Geometry check sheet. Reference: the model listing, model coordinates, mm. A direction names the side the tool comes from. Give positions to 0.01 mm unless a question says otherwise; leave off trailing zeros. Write item = value, one per line. Start each with the question number.
1. Depth check by flat-ended pin: P1, Ø4, axis at x = -1.5, z = -34, coming from the -Y side; P2, Ø1.3, axis at y = -2, z = -67, coming from the +X side; P3, Ø1.3, axis at x = -1.5, z = -132.5, coming from the +Y side; P4, Ø0.8, axis at y = -1, z = -51, coming from the -X side. Enter the tip coordinate at first touch or a pass-through.
2. Thickness scan on line 1 along X through (y, z) = (4.25, -130.5); line 2 along Y through (x, z) = (9, -161); line 3 along Y through (x, z) = (7.75, -150.5). Record the ranges inside material, lowest first.
3. Mould release check, pull along Y, two halves, no side actions. Record for faces 3 (the flat face through (6, 10, -99)), 4 (the flat face through (5.55, -4.49, -98.6)), 5 (the flat face through (-6, -10, -99)): pulls with the +Y half, pulls with the -Y half, needs draft (parallel to the pull), parting line crosses it, or undercut.
4. Set-up check for faces 1 (the flat face through (10, -6, -99)), 2 (the flat face through (-5.51, -4.45, -98.6)): record each of +Z, -Z, +X, -X, +Y, -Y from which the full face is reachable in a straight line by a thin tool's end or side.
Autodesk Inventor part; units mm, degrees
ref_plane "to_frame_XY" through (0, 0, 0) normal (0, 0, 1) x (1, 0, 0)
ref_plane "to_frame_YZ" through (0, 0, 0) normal (1, 0, 0) x (0, 1, 0)
ref_plane "to_frame_ZX" through (0, 0, 0) normal (0, 1, 0) x (0, 0, 1)
sketch "Sketch_5" plane through (0, 0, 0) normal (0, 0, 1) x (1, 0, 0)
  arc A0 (-10, 3.3) -> (-9.7, 3) centre (-9.7, 3.3) ccw
  line L0 (-9.7, 3) -> (-8, 3)
  line L1 (-8, 3) -> (-8, 6)
  line L2 (-8, 6) -> (-7.0607, 6)
  line L3 (-7.0607, 6) -> (-4, 2.9393)
  line L4 (-4, 2.9393) -> (-4, 0.3)
  line L5 (-4, 0.3) -> (-3.7, 0)
  line L6 (-3.7, 0) -> (-4, -0.3)
  line L7 (-4, -0.3) -> (-4, -2.9393)
  line L8 (-4, -2.9393) -> (-7.0607, -6)
  line L9 (-7.0607, -6) -> (-8, -6)
  line L10 (-8, -6) -> (-8, -3)
  line L11 (-8, -3) -> (-9.7, -3)
  arc A1 (-9.7, -3) -> (-10, -3.3) centre (-9.7, -3.3) ccw
  line L12 (-10, -3.3) -> (-10, -9)
  arc A2 (-10, -9) -> (-9, -10) centre (-9, -9) ccw
  line L13 (-9, -10) -> (-3.3, -10)
  arc A3 (-3.3, -10) -> (-3, -9.7) centre (-3.3, -9.7) ccw
  line L14 (-3, -9.7) -> (-3, -8)
  line L15 (-3, -8) -> (-6, -8)
  line L16 (-6, -8) -> (-6, -7.0607)
  line L17 (-6, -7.0607) -> (-2.9393, -4)
  line L18 (-2.9393, -4) -> (-0.3, -4)
  line L19 (-0.3, -4) -> (0, -3.7)
  line L20 (0, -3.7) -> (0.3, -4)
  line L21 (0.3, -4) -> (2.9393, -4)
  line L22 (2.9393, -4) -> (6, -7.0607)
  line L23 (6, -7.0607) -> (6, -8)
  line L24 (6, -8) -> (3, -8)
  line L25 (3, -8) -> (3, -9.7)
  arc A4 (3, -9.7) -> (3.3, -10) centre (3.3, -9.7) ccw
  line L26 (3.3, -10) -> (9, -10)
  arc A5 (9, -10) -> (10, -9) centre (9, -9) ccw
  line L27 (10, -9) -> (10, -3.3)
  arc A6 (10, -3.3) -> (9.7, -3) centre (9.7, -3.3) ccw
  line L28 (9.7, -3) -> (8, -3)
  line L29 (8, -3) -> (8, -6)
  line L30 (8, -6) -> (7.0607, -6)
  line L31 (7.0607, -6) -> (4, -2.9393)
  line L32 (4, -2.9393) -> (4, -0.3)
  line L33 (4, -0.3) -> (3.7, 0)
  line L34 (3.7, 0) -> (4, 0.3)
  line L35 (4, 0.3) -> (4, 2.9393)
  line L36 (4, 2.9393) -> (7.0607, 6)
  line L37 (7.0607, 6) -> (8, 6)
  line L38 (8, 6) -> (8, 3)
  line L39 (8, 3) -> (9.7, 3)
  arc A7 (9.7, 3) -> (10, 3.3) centre (9.7, 3.3) ccw
  line L40 (10, 3.3) -> (10, 9)
  arc A8 (10, 9) -> (9, 10) centre (9, 9) ccw
  line L41 (9, 10) -> (3.3, 10)
  arc A9 (3.3, 10) -> (3, 9.7) centre (3.3, 9.7) ccw
  line L42 (3, 9.7) -> (3, 8)
  line L43 (3, 8) -> (6, 8)
  line L44 (6, 8) -> (6, 7.0607)
  line L45 (6, 7.0607) -> (2.9393, 4)
  line L46 (2.9393, 4) -> (0.3, 4)
  line L47 (0.3, 4) -> (0, 3.7)
  line L48 (0, 3.7) -> (-0.3, 4)
  line L49 (-0.3, 4) -> (-2.9393, 4)
  line L50 (-2.9393, 4) -> (-6, 7.0607)
  line L51 (-6, 7.0607) -> (-6, 8)
  line L52 (-6, 8) -> (-3, 8)
  line L53 (-3, 8) -> (-3, 9.7)
  arc A10 (-3, 9.7) -> (-3.3, 10) centre (-3.3, 9.7) ccw
  line L54 (-3.3, 10) -> (-9, 10)
  arc A11 (-9, 10) -> (-10, 9) centre (-9, 9) ccw
  line L55 (-10, 9) -> (-10, 3.3)
  circle A12 centre (0, 0) radius 2.1
extrude "Extrusion1" add sketch "Sketch_5" against normal blind 1000
ref_plane "to_frame_XY" through (0, 0, 0) normal (0, 0, 1) x (1, 0, 0)
ref_plane "to_frame_YZ" through (0, 0, 0) normal (1, 0, 0) x (0, 1, 0)
ref_plane "to_frame_ZX" through (0, 0, 0) normal (0, 1, 0) x (0, 0, 1)
sketch "Sketch2" plane through (-10, -3.3, -1000) normal (-1, 0, 0) x (0, 0, 1)
  line L0 (-197.6604, -150.7885) -> (800, -150.7885)
  line L1 (800, -150.7885) -> (800, 147.9074)
  line L2 (800, 147.9074) -> (-197.6604, 147.9074)
  line L3 (-197.6604, 147.9074) -> (-197.6604, -150.7885)
  point P0 (1000, 3.3)
  dimension "d3" = 200
extrude "Extrusion2" cut sketch "Sketch2" against normal through all
equation "\"d0\" = L"
equation "\"L\" = 1000"
properties part number "2020 Extrusion 122mm"
Answers:
q1.P1 = -10
q1.P2 = 4
q1.P3 = 4
q1.P4 = -4
q2.line_1 = -10 to -8, -5.31 to -3.19, 3.19 to 5.31, 8 to 10
q2.line_2 = -10 to -3, 3 to 10
q2.line_3 = -10 to -6, 6 to 10
q3.face_3 = pulls with the +Y half
q3.face_4 = undercut
q3.face_5 = pulls with the -Y half
q4.face_1 = +Z, -Z, +X, +Y, -Y
q4.face_2 = +Z, -Z
